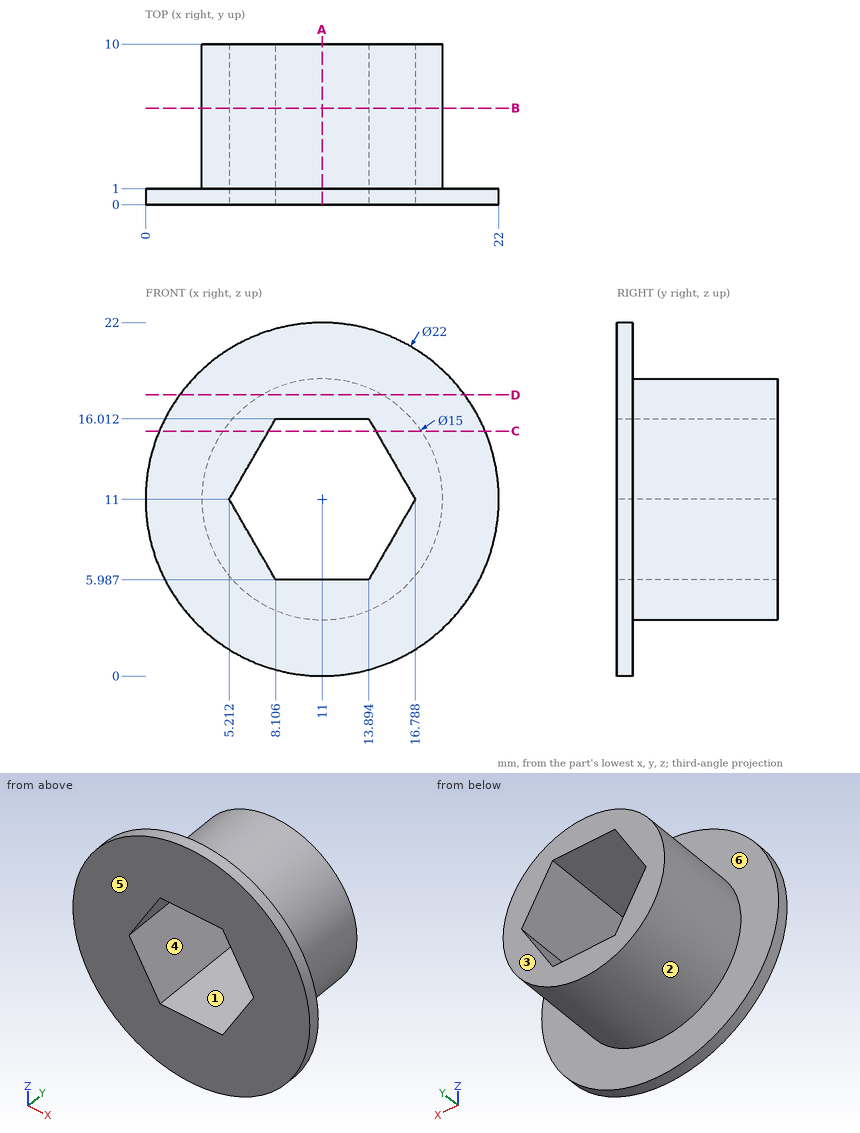
Drawing for the job (mm, zero at the part's lowest x, y, z). A direction names the side the tool comes from. Give positions to 0.01 mm unless a question says otherwise; leave off trailing zeros. Order: outer loops, then holes, each group sorted by start corner. A loop starts at its lowest first (then second) coordinate and runs counter-clockwise, first axis right, second up. Notation, with made-up numbers: M 79,6.25 L 117,6.25 A24 ccw 117,28.25 Z; hole C 49,0.25 d3. An arc over 180 degrees is marked long. Use a Markdown table: item, result. Add a question column.
(1) Probe line 1 along Y through (x, z) = (1, 8.5); line 2 along Z through (x, y) = (11.75, 5.5); line 3 along X through (y, z) = (9.5, 8) (1 decimal). List the from-to ranges inside material, lowest first. Write a range as [from, to].
(2) Mould opens along X. For the marked faces 1, 2 and 3 say: +X half, -X half, draft (parallel to the pull), parting line (faces both ways), or undercut.
(3) Saw through at B-B, the plane y = 6. Give the cut face in (x, z).
(4) 3-axis set-ups, long thin cutter, end or side, ignore diameter. For the marked faces 4, 5 and 6: which of +Z, -Z, +X, -X, +Y, -Y reach the whole face in a straight line?
(5) Drop flat-ended pins along their axis: P1, Ø1, axis at x = 10, y = 4.5, coming from the -Z side; P2, Ø11, axis at x = 14.5, z = 11, coming from the +Y side; P3, Ø4, axis at x = 8, y = 4, coming from the +Z side; P4, Ø1.5, axis at y = 6, z = 14.5, coming from the +X side. Give the stop position or say it passes through.
(6) Saw through at C-C, the plane z = 15.25. Give the cut face in (x, y) (1 decimal).
(7) Saw through at A-A, the plane x = 11. Give the cut face in (y, z).
(8) Saw through at D-D, the plane z = 17.5. Give the cut face in (x, y) (1 decimal).
Answer key:
| question | item | result |
|---|---|---|
| 1 | line 1 | [0, 1] |
| 1 | line 2 | [3.54, 5.99], [16.01, 18.46] |
| 1 | line 3 | [4.1, 6.9], [15.1, 17.9] |
| 2 | face 1 | undercut |
| 2 | face 2 | parting line |
| 2 | face 3 | draft |
| 3 | outline | C 11,11 d15; hole M 5.21,11 L 8.11,5.99 L 13.89,5.99 L 16.79,11 L 13.89,16.01 L 8.11,16.01 Z |
| 4 | face 4 | +Y, -Y |
| 4 | face 5 | +Z, -Z, +X, -X, -Y |
| 4 | face 6 | +Y |
| 5 | P1 | z = 3.52 |
| 5 | P2 | y = 10 |
| 5 | P3 | z = 18.43 |
| 5 | P4 | x = 17.98 |
| 6 | outline | M 0.9,0 L 7.7,0 L 7.7,10 L 4.8,10 L 4.8,1 L 0.9,1 Z; M 14.3,0 L 21.1,0 L 21.1,1 L 17.2,1 L 17.2,10 L 14.3,10 Z |
| 7 | outline | M 0,0 L 1,0 L 1,3.5 L 10,3.5 L 10,5.99 L 0,5.99 Z; M 0,16.01 L 10,16.01 L 10,18.5 L 1,18.5 L 1,22 L 0,22 Z |
| 8 | outline | M 2.1,0 L 19.9,0 L 19.9,1 L 14.7,1 L 14.7,10 L 7.3,10 L 7.3,1 L 2.1,1 Z |
